The listing builds one solid part. Answer for the finished solid, in the listing's coordinates (mm). A direction names the side the tool comes from. Give positions to 0.01 mm unless a question says otherwise; leave off trailing zeros. Order: outer loops, then holes, each group sorted by start corner. A loop starts at its lowest first (then second) coordinate and runs counter-clockwise, first axis right, second up. Notation, with made-up numbers: (45.25, 18) - (69.25, 18) arc R34 ccw to (69.25, 51) - close; hole circle Ø10 at (45, -36). An arc over 180 degrees is marked (long way). Answer as CSV lines item,"result". Start each with the question number.
1. Section C-C on x = 20 is taken. Give the vertices of the cut face in (y, z), and give its area (3 significant figures).
2. Section A-A on z = 0 is taken. Give the vertices of the cut face in (x, y), and give its area (3 significant figures).
3. Flat-ended cylindrical pins translate along their axes: pin 1 (2 mm diameter, centred on y = 45.5, z = 4, fed in from +X); pin 2 (5 mm diameter, centred on y = 25.5, z = -0.5, fed in from -X); pin 3 (5 mm diameter, centred on x = -20.5, z = -1.5, fed in from +Y). Find the tip coordinate at first contact, or state that the pin passes through.
4. Consider line 1 along X through (y, z) = (6, 0); line 2 along Y through (x, z) = (0, 2); line 3 along Y through (x, z) = (23.5, 4). Determine where each line is inside the solid, lowest interval first. Write a range as [from, to].
5. Which of the six approach directions +Z, -Z, +X, -X, +Y, -Y give full straight-line access (tool end or side, diameter ignored) to faces 1 (the flat face through (-22.3, 10, -0.1)), 2 (the flat face through (0, 21, 5))?
6. Determine the mould class of faces 3 (the flat face through (17.7, 10, -0.1)), 4 (the flat face through (15, 32, 0)), 5 (the cylindrical face through (22, 5, 0)) for opening direction X: +X half, -X half, draft (parallel to the pull), parting line (faces both ways), or undercut.
7. Section B-B on y = 40 is taken. Give the vertices of the cut face in (x, z).
8. Section D-D on z = 4 is taken. Give the vertices of the cut face in (x, y).
from build123d import *

# Parameters (mm, degrees)
SKETCH1_W           = 50
SKETCH1_H           = 10
SKETCH1_R           = 2
BOSS_EXTRUDE1_DEPTH = 10
SKETCH4_W           = 30
SKETCH4_H           = 10
BOSS_EXTRUDE3_DEPTH = 45
SKETCH5_R           = 4
CUT_EXTRUDE1_DEPTH  = 45


with BuildPart() as part:
    # Sketch1 → Boss-Extrude1 (new body)
    with BuildSketch(Plane(origin=(0, 0, 0), x_dir=(1, 0, 0), z_dir=(0, 1, 0))):
        Rectangle(SKETCH1_W, SKETCH1_H)
        with Locations(Location((-20, 0, 0), (0, 0, 270))):
            Circle(SKETCH1_R, mode=Mode.SUBTRACT)
        with Locations(Location((20, 0, 0), (0, 0, 270))):
            Circle(SKETCH1_R, mode=Mode.SUBTRACT)
    extrude(amount=BOSS_EXTRUDE1_DEPTH)

    # Sketch4 → Boss-Extrude3 (add)
    with BuildSketch(Plane(origin=(0, 10, 0), x_dir=(1, 0, 0), z_dir=(0, 1, 0))):
        Rectangle(SKETCH4_W, SKETCH4_H)
    extrude(amount=BOSS_EXTRUDE3_DEPTH)

    # Sketch5 → Cut-Extrude1 (cut)
    with BuildSketch(Plane.XY.offset(5)):
        with Locations((0, 40)):
            Circle(SKETCH5_R)
    extrude(amount=-CUT_EXTRUDE1_DEPTH, mode=Mode.SUBTRACT)


solid = part.part
Checks:
1,outline,"(0, -5) - (10, -5) - (10, -2) - (0, -2) - close; (0, 2) - (10, 2) - (10, 5) - (0, 5) - close"
1,area,"60.0 mm²"
2,outline,"(-25, 0) - (-22, 0) - (-22, 10) - (-25, 10) - close; (-18, 0) - (18, 0) - (18, 10) - (15, 10) - (15, 55) - (-15, 55) - (-15, 10) - (-18, 10) - close; (22, 0) - (25, 0) - (25, 10) - (22, 10) - close; hole circle Ø8 at (0, 40)"
2,area,"1,720 mm²"
3,pin 1,"stops at x = 15"
3,pin 2,"stops at x = -15"
3,pin 3,"stops at y = 10"
4,line 1,"x = [-25, -22], [-18, 18], [22, 25]"
4,line 2,"y = [0, 36], [44, 55]"
4,line 3,"y = [0, 10]"
5,face 1,"+Z, -Z, -X, +Y"
5,face 2,"+Z, +X, -X, +Y, -Y"
6,face 3,"draft"
6,face 4,"+X half"
6,face 5,"undercut"
7,outline,"(-15, -5) - (-4, -5) - (-4, 5) - (-15, 5) - close; (4, -5) - (15, -5) - (15, 5) - (4, 5) - close"
8,outline,"(-25, 0) - (25, 0) - (25, 10) - (15, 10) - (15, 55) - (-15, 55) - (-15, 10) - (-25, 10) - close; hole circle Ø8 at (0, 40)"
